Could you check a few things on this model? Use its own coordinates, in mm. Give positions to 0.01 mm unless a question says otherwise; leave off trailing zeros. Loops run counter-clockwise (first coordinate to the right, second up) from the corner with the lowest first, then second, coordinate; pieces in that order, holes last. Notation, with made-up numbers: (85, -21.5) - (140, -21.5) arc R35 ccw to (140, 14.5) - close; hole circle Ø11 at (24.25, 66). An arc over 180 degrees is marked (long way). Use CSV: the item, a comma, the result in double quotes.
from build123d import *

# Parameters (mm, degrees)
F1_DEPTH = 50.8
F2_SIZE  = 20


with BuildPart() as f1:
    # F0 (on Top) → F1 (new body)
    with BuildSketch(Plane.XY):
        Polygon((13.774368, -27.66192), (30.564563, 4.552199), (5.115571, 30.475334), (-27.402966, 14.282593), (-22.051536, -21.648205), align=None)
    extrude(amount=F1_DEPTH)

    # F2
    f2_edges = [f1.edges().sort_by_distance(p)[0] for p in [
        (-4.138584, -24.655063, 50.8),
        (22.169465, -11.554861, 50.8),
        (17.840067, 17.513766, 50.8),
        (-11.143697, 22.378964, 50.8),
        (-24.727251, -3.682806, 50.8),
    ]]
    chamfer(f2_edges, length=F2_SIZE)


solid = f1.part
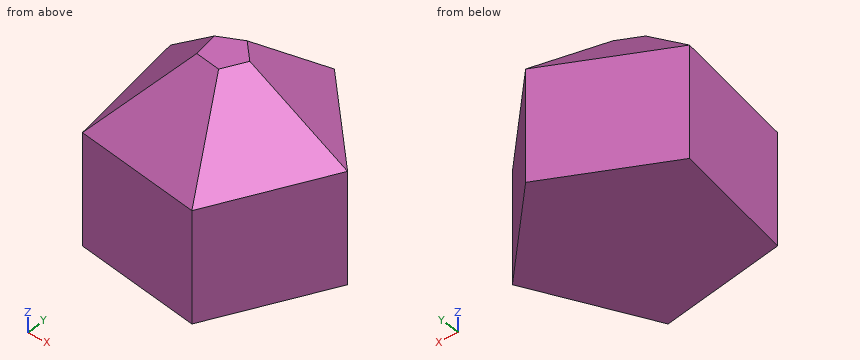
1) Suppose I cut it at A-A (z = 11). Please give me the cut outline in (x, y).
Answer below:
outline,"(-27.4, 14.28) - (-22.05, -21.65) - (13.77, -27.66) - (30.56, 4.55) - (5.12, 30.48) - close"
2) I'm going to push flat-ended pins straight in: P1, Ø12, axis at x = 13.5, y = -6.5, coming from the +Z side; P2, Ø5, axis at x = 6, z = 26, coming from the +Y side; P3, Ø1, axis at x = 1.5, z = 44, coming from the -Y side; P4, Ø1.5, axis at x = 1, y = -11, coming from the -Z side. Where does each tip first touch, or does it pass through?
Answer below:
P1,"stops at z = 46.82"
P2,"stops at y = 30.48"
P3,"stops at y = -12.73"
P4,"stops at z = 0"
3) I need wall thicknesses on line 1 along Z through (x, y) = (11, 2); line 2 along Z through (x, y) = (-10, 9); line 3 along X through (y, z) = (24.5, 17.5). Which ranges of each line are inside material? Lowest first, please.
Answer below:
line 1,"z = 0 to 46.55"
line 2,"z = 0 to 43.29"
line 3,"x = -6.88 to 10.98"
4) Suppose I cut it at B-B (x = -8.5). Please give me the cut outline in (y, z).
Answer below:
outline,"(-23.92, 0) - (23.7, 0) - (23.7, 30.8) - (4.43, 48.05) - (-8.34, 46.16) - (-23.92, 30.8) - close"
5) Suppose I cut it at C-C (y = 21.5). Please give me the cut outline in (x, z), plus the area to 3 significant figures.
Answer below:
outline,"(-12.91, 0) - (13.93, 0) - (13.93, 30.8) - (3.61, 38.16) - (-12.91, 30.8) - close"
area,"925 mm2"
6) Suppose I cut it at D-D (x = -20). Please give me the cut outline in (y, z).
Answer below:
outline,"(-21.99, 0) - (17.97, 0) - (17.97, 30.8) - (10.42, 37.55) - (-19.63, 33.13) - (-21.99, 30.8) - close"
